Study the drawing (mm; zero at the part's minimum x, y, z) and answer. A direction names the side the tool comes from. Give positions to 0.01 mm unless a question says otherwise; leave off trailing zeros. Write each loop counter-clockwise with the first axis right and the second up, starting at its lowest first coordinate (ties: lowest second). Pieces come first, ordered by that corner, then holes.
1) Find section B-B (x = 26). Determine the outline of the cut face in (y, z), plus the area to 3 significant figures.
2) Determine the mould class of the marked faces 1, 2 and 3 for opening direction X: pulls with the +X half, pulls with the -X half, needs draft (parallel to the pull), parting line crosses it, or undercut.
3) A tool of negligible diameter and unlimited length cuts with its end or side. For the marked faces 4 and 5, from which of +Z, -Z, +X, -X, +Y, -Y can it reach the whole face along a straight path? Write none if from no direction.
4) Straight lines are drawn through the part: probe 1 along Z at (x, y) = (20, 5.75); probe 2 along Y at (x, z) = (23.5, 35); probe 3 along Z at (x, y) = (6.5, 8). For each, find the intervals that lie inside material, in ascending order.
5) Find section C-C (z = 20). Determine the outline of the cut face in (x, y).
6) Given pin 1 Ø3 at (x, y) = (7, 6) entering from -Z; pin 2 Ø1.5 at (x, z) = (10, 19.5) entering from -Y, each flat-ended and moving along its own axis, determine where each tip first touches the part or whether it passes through.
7) Find section A-A (y = 3.25). Determine the outline of the cut face in (x, z).
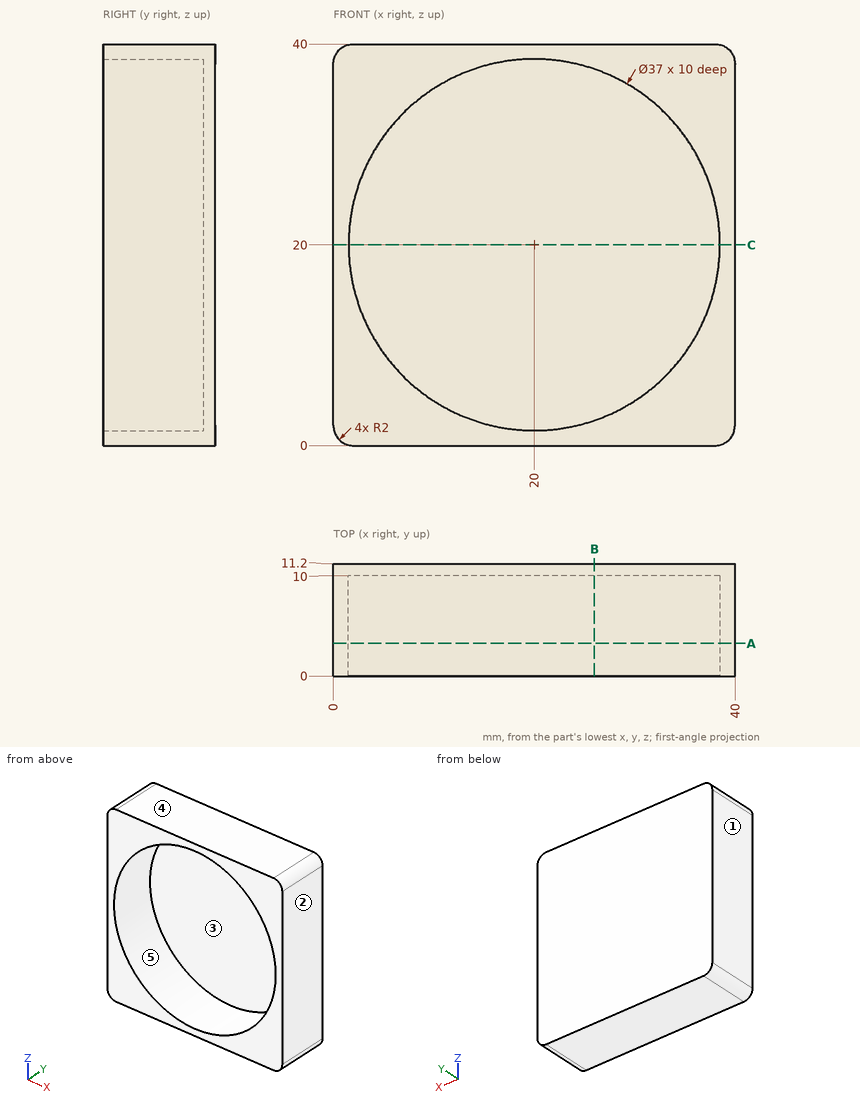
Results:
1. outline: (0, 0) - (11.2, 0) - (11.2, 40) - (0, 40) - (0, 37.5) - (10, 37.5) - (10, 2.5) - (0, 2.5) - close
1. area: 98.0 mm2
2. face 1: pulls with the -X half
2. face 2: pulls with the +X half
2. face 3: undercut
3. face 4: +Z, +X, -X, +Y, -Y
3. face 5: -Y
4. probe 1: z = 0 to 1.5, 38.5 to 40
4. probe 2: y = 10 to 11.2
4. probe 3: z = 0 to 7.35, 32.65 to 40
5. outline: (0, 0) - (1.5, 0) - (1.5, 10) - (38.5, 10) - (38.5, 0) - (40, 0) - (40, 11.2) - (0, 11.2) - close
6. pin 1: stops at z = 0
6. pin 2: stops at y = 10
7. outline: (0, 2) arc R2 ccw to (2, 0) - (38, 0) arc R2 ccw to (40, 2) - (40, 38) arc R2 ccw to (38, 40) - (2, 40) arc R2 ccw to (0, 38) - close; hole circle Ø37 at (20, 20)
